Drawing for the job (mm, zero at the part's lowest x, y, z). Round coordinates to 2 decimals unless told otherwise and drop trailing zeros. Write each loop counter-clockwise with the first axis right and the second up, starting at its lowest first coordinate (ties: lowest second). Pieces come first, ordered by that corner, then holes.
Item 1: Wall check: probe 1 along Z at (x, y) = (5.5, 2.2) (1 decimal); probe 2 along Y at (x, z) = (1.5, 4.5) (1 decimal); probe 3 along Z at (x, y) = (4.75, 4.1). Give the ranges that are in metal, low to high.
Item 2: Drop flat-ended pins along their axis: pin 1 Ø1 at (x, y) = (6, 4) entering from -Z (3 decimals); pin 2 Ø6 at (x, z) = (5.5, 5.5) entering from +Y; pin 3 Ø1 at (y, z) = (3.5, 1.5) entering from -X (1 decimal). Give the stop position or say it passes through.
Item 3: Mould opens along X. For the marked faces 1, 2 and 3 say: +X half, -X half, draft (parallel to the pull), parting line (faces both ways), or undercut.
Item 4: Band-saw the part on C-C, the plane y = 1.4. Write the cut outline in (x, z).
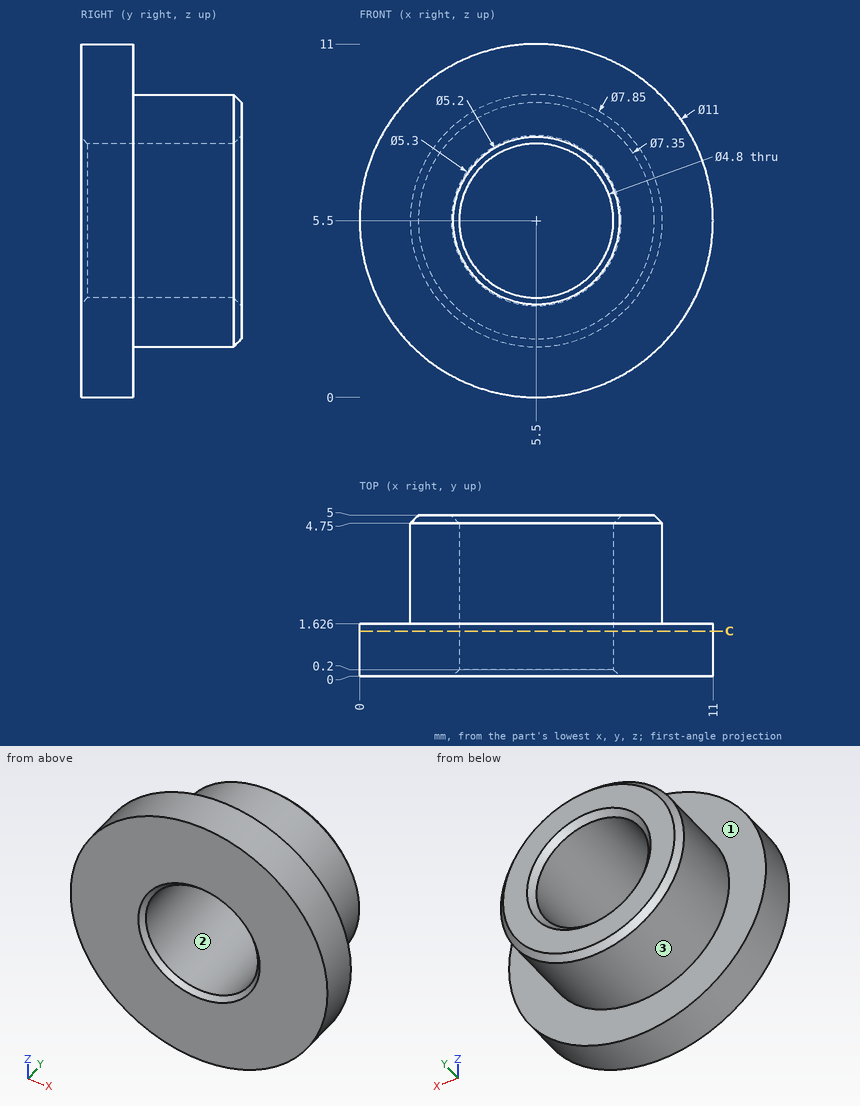
Results:
1. probe 1: z = 1.6 to 3.1, 7.9 to 9.4
1. probe 2: y = 0 to 1.6
1. probe 3: z = 1.65 to 3.22, 7.78 to 9.35
2. pin 1: stops at z = 1.575
2. pin 2: stops at y = 5
2. pin 3: stops at x = 3.7
3. face 1: draft
3. face 2: undercut
3. face 3: parting line
4. outline: circle Ø11 at (5.5, 5.5); hole circle Ø4.8 at (5.5, 5.5)
